```python
from build123d import *

# Parameters (mm, degrees)
SKETCH2_W           = 10
SKETCH2_H           = 10
BOSS_EXTRUDE1_DEPTH = 400
SKETCH3_R           = 15
BOSS_EXTRUDE2_DEPTH = 10
SKETCH4_R           = 10
CUT_EXTRUDE1_DEPTH  = 10
CUT_EXTRUDE2_START  = 15
SKETCH5_OUTSIDE_W   = 237.072
SKETCH5_OUTSIDE_H   = 237.072
SKETCH5_OUTSIDE_W_2 = 6.67
SKETCH5_OUTSIDE_H_2 = 6.67
CUT_EXTRUDE2_DEPTH  = 400
CUT_EXTRUDE2_TAPER  = 7
FILLET1_R           = 0.5
FILLET2_R           = 5


with BuildPart() as part:
    # Sketch1 → Revolve1 (revolve)
    with BuildSketch(Plane.XY):
        with BuildLine():
            Line((0, 24), (0, -24))
            ThreePointArc((0, -24), (24, 0), (0, 24))
        make_face()
    revolve(axis=Axis((0, 24, 0), (0, -1, 0)))

    # Sketch2 → Boss-Extrude1 (add)
    with BuildSketch(Plane.XY):
        Rectangle(SKETCH2_W, SKETCH2_H)
    extrude(amount=BOSS_EXTRUDE1_DEPTH)

    # Sketch3 → Boss-Extrude2 (add)
    with BuildSketch(Plane(origin=(0, 5, 0), x_dir=(1, 0, 0), z_dir=(0, 1, 0))):
        with Locations((0, -400)):
            Circle(SKETCH3_R)
    extrude(amount=-BOSS_EXTRUDE2_DEPTH)

    # Sketch4 → Cut-Extrude1 (cut)
    with BuildSketch(Plane(origin=(0, 5, 0), x_dir=(1, 0, 0), z_dir=(0, 1, 0))):
        with Locations(Location((0, -400, 0), (0, 0, 270))):
            Circle(SKETCH4_R)
    extrude(amount=-CUT_EXTRUDE1_DEPTH, mode=Mode.SUBTRACT)

    # Sketch5 outside → Cut-Extrude2 (cut)
    with BuildSketch(Plane.XY.offset(CUT_EXTRUDE2_START)):
        Rectangle(SKETCH5_OUTSIDE_W, SKETCH5_OUTSIDE_H)
        Rectangle(SKETCH5_OUTSIDE_W_2, SKETCH5_OUTSIDE_H_2, mode=Mode.SUBTRACT)
    extrude(amount=CUT_EXTRUDE2_DEPTH, taper=CUT_EXTRUDE2_TAPER, mode=Mode.SUBTRACT)

    # Fillet1
    fillet1_edges = [part.edges().sort_by_distance(p)[0] for p in [
        (3.335, 0, 15),
        (0, 3.335, 15),
        (-3.335, 0, 15),
        (0, -3.335, 15),
    ]]
    fillet(fillet1_edges, radius=FILLET1_R)

    # Fillet2
    fillet2_edges = [part.edges().sort_by_distance(p)[0] for p in [
        (0, -18.734993995, 15),
    ]]
    fillet(fillet2_edges, radius=FILLET2_R)


solid = part.part
```
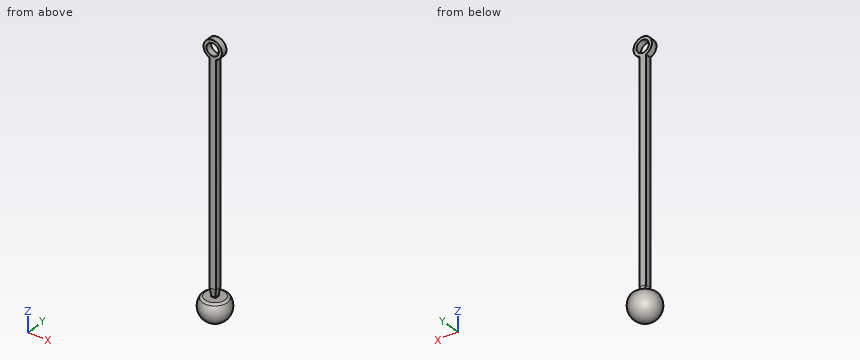
Source: CAD feature listing. Evaluate the final solid. Frame: model axes, mm. Coordinates: 2 decimals unless noted, no trailing zeros. Write each loop counter-clockwise with the first axis right and the second up, starting at its lowest first coordinate (ties: lowest second). Pieces come first, ordered by that corner, then holes. Notation, with made-up numbers: (2.5, -5.5) -> (23.5, -5.5) arc R12 ccw to (23.5, 13.5) -> close; hole circle Ø3 at (60.25, -17.5). An arc over 180 degrees is marked (long way). Return JSON: item names as keys, results as strings. Group by question number.
1) Section query B-B, the plane z = 294. Return loops of the section in (x, y), plus the area to 3 significant figures.
2) Contact query for flat-ended pins moving along their axis: P1, Ø8, axis at x = -7, y = -16.5, coming from the +Z side; P2, Ø11, axis at y = -0.5, z = 268, coming from the -X side; P3, Ø10, axis at y = -7.5, z = 274.5, coming from the +X side. Output: stop coordinate, or through.
3) Ray query, line 1 along X through (y, z) = (0, 400); line 2 along X through (y, z) = (-1, 370). Return the intervals inside material, ascending.
4) Section query A-A, the plane z = 400. Return loops of the section in (x, y), plus the area to 3 significant figures.
From the geometry:
{
 "1": {"outline": "(-5, -5) -> (5, -5) -> (5, 5) -> (-5, 5) -> close", "area": "100 mm²"},
 "2": {"P1": "z = 15", "P2": "x = -5", "P3": "x = 5"},
 "3": {"line 1": "-15 to -10, 10 to 15", "line 2": "-5 to 5"},
 "4": {"outline": "(-15, -5) -> (-10, -5) -> (-10, 5) -> (-15, 5) -> close; (10, -5) -> (15, -5) -> (15, 5) -> (10, 5) -> close", "area": "100 mm²"}
}
